Read the model definition and answer for the solid it produces. Units are mm, in the model's axes. A direction names the side the tool comes from. Coordinates: 2 decimals unless noted, no trailing zeros. Write each loop counter-clockwise with the first axis right and the second up, starting at its lowest first coordinate (ties: lowest second). Pieces come first, ordered by that corner, then holes. Notation, with made-up numbers: (10.5, -32.5) -> (30.5, -32.5) arc R24 ccw to (30.5, 2.5) -> close; hole circle Ø7 at (6, 23.5). An arc over 180 degrees is marked (long way). Answer in a Markdown table with one row per item. Add a question column.
Item 1: Section C-C on x = 43 is taken. Write down the section's boundary in (y, z).
Item 2: Which of the six approach directions +Z, -Z, +X, -X, +Y, -Y give full straight-line access (tool end or side, diameter ignored) to faces 1 (the face through (18, 16, 35)), 2 (the face through (-81, 16, 17)), 3 (the face through (-16, 45, 14))?
Item 3: Straight lines are drawn through the part: line 1 (Z direction, x = -15, y = 41.75); line 2 (X direction, y = 60, z = -25.5); line 3 (X direction, y = 54.5, z = -31). For each, find the intervals that lie inside material, in ascending order. Write a range as from..to.
Item 4: For a pull along Z with two mould halves and no side action, classify faces 4 (the face through (67, 145, -9)), 5 (the face through (-14.34, 37.61, 14.64)), 6 (the face through (50, 16, 17)), 7 (the face through (75, 106, -10)) as +Z half, -Z half, draft (parallel to the pull), parting line (faces both ways), or undercut.
Item 5: Given pin 1 Ø1.5 at (x, z) = (67, -8.5) entering from -Y; pin 2 Ø6 at (y, z) = (45.5, -30.5) entering from -X; pin 3 Ø16.5 at (y, z) = (24, 43) entering from -X; pin 4 Ø16 at (x, y) = (53.5, 95) entering from +Z, each flat-ended and moving along its own axis, determine where each tip first touches the part or whether it passes through.
Item 6: Section D-D on y = 51 is taken. Write down the section's boundary in (x, z), then the cut area to 3 significant figures.
Item 7: Section B-B on z = -4 is taken. Write down the section's boundary in (x, y).
Item 8: Section A-A on y = 142 is taken. Write down the section's boundary in (x, z).
```python
from build123d import *

# Parameters (mm, degrees)
SKETCH1_W            = 240
SKETCH1_H            = 100
BOSS_EXTRUDE1_DEPTH  = 15
SKETCH5_W            = 15
SKETCH5_H            = 50
BOSS_EXTRUDE4_DEPTH  = 180
SKETCH12_W           = 150
SKETCH12_H           = 50
BOSS_EXTRUDE7_DEPTH  = 30
FILLET1_R            = 5
FILLET4_R            = 5
FILLET10_R           = 5
BOSS_EXTRUDE8_DEPTH  = 30
SKETCH17_R           = 15
CUT_EXTRUDE1_DEPTH   = 15
SKETCH18_W           = 15
SKETCH18_H           = 15
CUT_EXTRUDE3_DEPTH   = 15
FILLET11_R           = 5
FILLET12_R           = 5
FILLET13_R           = 5
FILLET14_R           = 5
BOSS_EXTRUDE10_DEPTH = 150
FILLET19_R           = 1.5
FILLET20_R           = 1.5
SKETCH24_W           = 75
SKETCH24_H           = 150
BOSS_EXTRUDE11_DEPTH = 5
FILLET23_R           = 2
FILLET24_R           = 2
FILLET25_R           = 10
FILLET26_R           = 10
FILLET27_R           = 10
FILLET28_R           = 10
SKETCH25_W           = 5
SKETCH25_H           = 20
CUT_EXTRUDE4_DEPTH   = 271.046292328


with BuildPart() as part:
    # Sketch1 → Boss-Extrude1 (new body)
    with BuildSketch(Plane(origin=(0, 0, 0), x_dir=(1, 0, 0), z_dir=(0, 1, 0))):
        Rectangle(SKETCH1_W, SKETCH1_H)
    extrude(amount=BOSS_EXTRUDE1_DEPTH)

    # Sketch5 → Boss-Extrude4 (add)
    with BuildSketch(Plane(origin=(0, 15, 0), x_dir=(1, 0, 0), z_dir=(0, 1, 0))):
        with Locations((-97.5, 10)):
            Rectangle(SKETCH5_W, SKETCH5_H)
        with Locations((67.5, 10)):
            Rectangle(SKETCH5_W, SKETCH5_H)
    extrude(amount=BOSS_EXTRUDE4_DEPTH)

    # Sketch12 → Boss-Extrude7 (add)
    with BuildSketch(Plane(origin=(0, 15, 0), x_dir=(1, 0, 0), z_dir=(0, 1, 0))):
        with Locations((-15, 10)):
            Rectangle(SKETCH12_W, SKETCH12_H)
    extrude(amount=BOSS_EXTRUDE7_DEPTH)

    # Fillet1
    fillet1_edges = [part.edges().sort_by_distance(p)[0] for p in [
        (-105, 15, -10),
    ]]
    fillet(fillet1_edges, radius=FILLET1_R)

    # Fillet4
    fillet4_edges = [part.edges().sort_by_distance(p)[0] for p in [
        (-17.5, 15, -35),
    ]]
    fillet(fillet4_edges, radius=FILLET4_R)

    # Fillet10
    fillet10_edges = [part.edges().sort_by_distance(p)[0] for p in [
        (75, 15, -12.5),
    ]]
    fillet(fillet10_edges, radius=FILLET10_R)

    # Sketch15 → Boss-Extrude8 (add)
    with BuildSketch(Plane(origin=(0, 15, 0), x_dir=(1, 0, 0), z_dir=(0, 1, 0))):
        Polygon((-15, -15), (16, -15), (16, -50), (-46, -50), (-46, -15), align=None)
    extrude(amount=BOSS_EXTRUDE8_DEPTH)

    # Sketch17 → Cut-Extrude1 (cut)
    with BuildSketch(Plane(origin=(0, 45, 0), x_dir=(1, 0, 0), z_dir=(0, 1, 0))):
        with Locations(Location((-15, -29.627354627, 0), (0, 0, 270))):
            Circle(SKETCH17_R)
    extrude(amount=-CUT_EXTRUDE1_DEPTH, mode=Mode.SUBTRACT)

    # Sketch18 → Cut-Extrude3 (cut)
    with BuildSketch(Plane.XY.offset(50)):
        with Locations((-17.79206598, 25.674800875)):
            Rectangle(SKETCH18_W, SKETCH18_H)
    extrude(amount=-CUT_EXTRUDE3_DEPTH, mode=Mode.SUBTRACT)

    # Fillet11
    fillet11_edges = [part.edges().sort_by_distance(p)[0] for p in [
        (48, 15, 15),
    ]]
    fillet(fillet11_edges, radius=FILLET11_R)

    # Fillet12
    fillet12_edges = [part.edges().sort_by_distance(p)[0] for p in [
        (-78, 15, 15),
    ]]
    fillet(fillet12_edges, radius=FILLET12_R)

    # Fillet13
    fillet13_edges = [part.edges().sort_by_distance(p)[0] for p in [
        (16, 15, 35),
        (16, 32.5, 15),
        (16, 16.464466094, 16.464466094),
    ]]
    fillet(fillet13_edges, radius=FILLET13_R)

    # Fillet14
    fillet14_edges = [part.edges().sort_by_distance(p)[0] for p in [
        (-46, 32.5, 15),
        (-46, 15, 35),
        (-46, 16.464466094, 16.464466094),
    ]]
    fillet(fillet14_edges, radius=FILLET14_R)

    # Sketch23 → Boss-Extrude10 (add)
    with BuildSketch(Plane.ZY.offset(-60)):
        Polygon((-9.66, 45), (-14.66, 45), (-13.41, 55), (-10.91, 55), align=None)
    extrude(amount=BOSS_EXTRUDE10_DEPTH)

    # Fillet19
    fillet19_edges = [part.edges().sort_by_distance(p)[0] for p in [
        (-15, 55, -10.91),
    ]]
    fillet(fillet19_edges, radius=FILLET19_R)

    # Fillet20
    # the kernel refuses this fillet: 1.5 mm, written as the material it takes off along each edge
    with BuildSketch(Plane(origin=(60, 55, -13.41), x_dir=(0, 0, 1), z_dir=(-1, 0, 0))) as fillet20_piece_1:
        with BuildLine():
            CenterArc((1.325104128, -1.492553597), FILLET20_R, 95.711432961, 77.16355069)
            Line((-0.163312687, -1.306501496), (-0.193081023, -1.302780453))
            Line((-0.193081023, -1.302780453), (-0.029768336, 0.003721042))
            Line((-0.029768336, 0.003721042), (0, 0.03))
            ThreePointArc((0, 0.03), (0.587913336, 0.03), (1.172841123, 0.029851072))
            Line((1.172841123, 0.029851072), (1.175826672, 0))
        make_face()
    extrude(amount=150, mode=Mode.SUBTRACT)

    # Sketch24 → Boss-Extrude11 (add)
    with BuildSketch(Plane(origin=(0, 0, -35), x_dir=(-1, 0, 0), z_dir=(0, 0, -1))):
        with Locations((52.5, 120)):
            Rectangle(SKETCH24_W, SKETCH24_H)
    extrude(amount=-BOSS_EXTRUDE11_DEPTH)

    # Fillet23
    fillet23_edges = [part.edges().sort_by_distance(p)[0] for p in [
        (-15, 45, -9.66),
    ]]
    fillet(fillet23_edges, radius=FILLET23_R)

    # Fillet24
    fillet24_edges = [part.edges().sort_by_distance(p)[0] for p in [
        (-15, 45, -14.66),
    ]]
    fillet(fillet24_edges, radius=FILLET24_R)

    # Fillet25
    fillet25_edges = [part.edges().sort_by_distance(p)[0] for p in [
        (120, 7.5, 50),
    ]]
    fillet(fillet25_edges, radius=FILLET25_R)

    # Fillet26
    fillet26_edges = [part.edges().sort_by_distance(p)[0] for p in [
        (120, 7.5, -50),
    ]]
    fillet(fillet26_edges, radius=FILLET26_R)

    # Fillet27
    fillet27_edges = [part.edges().sort_by_distance(p)[0] for p in [
        (-120, 7.5, 50),
    ]]
    fillet(fillet27_edges, radius=FILLET27_R)

    # Fillet28
    fillet28_edges = [part.edges().sort_by_distance(p)[0] for p in [
        (-120, 7.5, -50),
    ]]
    fillet(fillet28_edges, radius=FILLET28_R)

    # Sketch25 → Cut-Extrude4 (cut, through all)
    with BuildSketch(Plane.ZY.offset(-60)):
        with Locations((-9.462355362, 155)):
            Rectangle(SKETCH25_W, SKETCH25_H)
    extrude(amount=-CUT_EXTRUDE4_DEPTH, mode=Mode.SUBTRACT)


solid = part.part
```
Results below:
| question | item | result |
|---|---|---|
| 1 | outline | (0, -50) -> (15, -50) -> (15, -40) arc R5 cw to (20, -35) -> (45, -35) -> (45, -16.43) arc R2 cw to (46.75, -14.44) -> (53.69, -13.57) arc R1.5 ccw to (55, -12.23) arc R1.5 ccw to (53.69, -10.75) -> (46.75, -9.88) arc R2 cw to (45, -7.89) -> (45, 15) -> (20, 15) arc R5 cw to (15, 20) -> (15, 50) -> (0, 50) -> close |
| 2 | face 1 | +Z, +X, +Y |
| 2 | face 2 | +Z, -X, +Y |
| 2 | face 3 | +Z, +Y |
| 3 | line 1 | z = -35..14.63, 44.63..50 |
| 3 | line 2 | x = -105..-90, 60..75 |
| 3 | line 3 | x = -105..-15, 60..75 |
| 4 | face 4 | undercut |
| 4 | face 5 | undercut |
| 4 | face 6 | +Z half |
| 4 | face 7 | draft |
| 5 | pin 1 | stops at y = 0 |
| 5 | pin 2 | stops at x = -105 |
| 5 | pin 3 | stops at x = -48.37 |
| 5 | pin 4 | stops at z = 15 |
| 6 | outline | (-105, -35) -> (-15, -35) -> (-15, -30) -> (-90, -30) -> (-90, -13.91) -> (60, -13.91) -> (60, -35) -> (75, -35) -> (75, 15) -> (60, 15) -> (60, -10.41) -> (-90, -10.41) -> (-90, 15) -> (-105, 15) -> close |
| 6 | area | 2,400 mm2 |
| 7 | outline | (-120, 0) -> (120, 0) -> (120, 15) -> (80, 15) arc R5 cw to (75, 20) -> (75, 195) -> (60, 195) -> (60, 45) -> (-90, 45) -> (-90, 195) -> (-105, 195) -> (-105, 20) arc R5 cw to (-110, 15) -> (-120, 15) -> close |
| 8 | outline | (-105, -35) -> (-15, -35) -> (-15, -30) -> (-90, -30) -> (-90, 15) -> (-105, 15) -> close; (60, -35) -> (75, -35) -> (75, 15) -> (60, 15) -> close |
